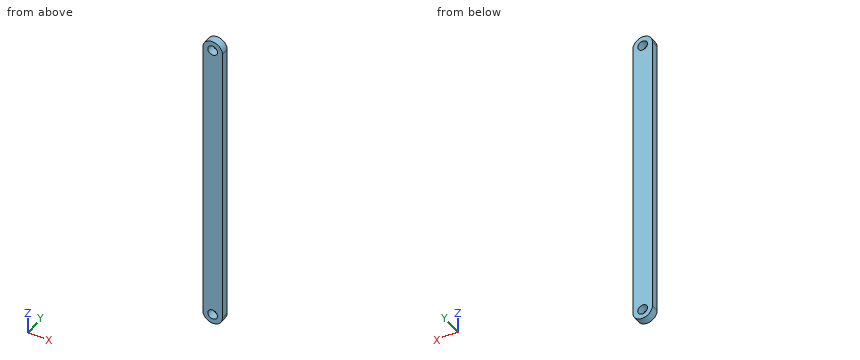
Autodesk Inventor part; units mm, degrees
ref_plane "YZ Plane" through (0, 0, 0) normal (1, 0, 0) x (0, 1, 0)
ref_plane "XZ Plane" through (0, 0, 0) normal (0, 1, 0) x (-1, 0, 0)
ref_plane "XY Plane" through (0, 0, 0) normal (0, 0, 1) x (1, 0, 0)
sketch "Schizzo1" plane through (0, 0, 0) normal (0, 1, 0) x (-1, 0, 0)
  line L0 (0, 0) -> (10, 0)
  line L1 (10, 0) -> (10, -150)
  line L2 (10, -150) -> (0, -150)
  line L3 (0, -150) -> (0, 0)
  dimension "d0" = 150
  dimension "d1" = 10
extrude "Estrusione1" add sketch "Schizzo1" along normal blind 4
sketch "Schizzo2" plane through (0, 4, 0) normal (0, 1, 0) x (1, 0, 0)
  line L0 (-10, 0) -> (0, 0)
  circle A0 centre (-5, 0) radius 5
  circle A1 centre (-5, 0) radius 2.5
  line L1 (0, 150) -> (-10, 150)
  circle A2 centre (-5, 150) radius 5
  circle A3 centre (-5, 150) radius 2.5
  point P0 (-7.5, 150)
  point P1 (-2.5, 150)
  point P2 (-2.5, 0)
  point P3 (-7.5, 0)
  dimension "d4" = 5
  dimension "d5" = 5
extrude "Estrusione2" add sketch "Schizzo2" against normal up to surface (4 mm away) contours A1 L0 A0 | L0 A0 A1 | A2 L1 A3 | L1 A3 A2
extrude "Estrusione3" cut sketch "Schizzo2" against normal blind 10 contours L0 A1 | A3 L1 picked at (-4.3762, 0.5526) picked at (-4.7045, 148.822)
properties part number "pod" material "Titanio"
Can you work these out from the model? Positions are in its coordinate system, mm. Round coordinates to 2 decimals unless told otherwise and drop trailing zeros. Order: outer loops, then holes, each group sorted by start corner. A loop starts at its lowest first (then second) coordinate and runs counter-clockwise, first axis right, second up.
(1) If we section it at B-B (y = 1.4): Please give me the cut outline in (x, z).
Results are:
outline: (-10, -150) arc R5 ccw to (0, -150) - (0, 0) arc R5 ccw to (-10, 0) - close; hole circle Ø5 at (-5, -150); hole circle Ø5 at (-5, 0)
(2) If I drill on L1, parallel to Z at x = -4.75, y = 3.05; L2, parallel to X at y = 2, z = -150; L3, parallel to Z at x = -6.75, y = 3.15, over which ranges is the centre line in solid material (lowest first)?
Results are:
L1: z = -154.99 to -152.49, -147.51 to -2.49, 2.49 to 4.99
L2: x = -10 to -7.5, -2.5 to 0
L3: z = -154.68 to -151.79, -148.21 to -1.79, 1.79 to 4.68
(3) If we section it at A-A (x = -5): Please give me the cut outline in (y, z).
Results are:
outline: (0, -155) - (4, -155) - (4, -152.5) - (0, -152.5) - close; (0, -147.5) - (4, -147.5) - (4, -2.5) - (0, -2.5) - close; (0, 2.5) - (4, 2.5) - (4, 5) - (0, 5) - close
